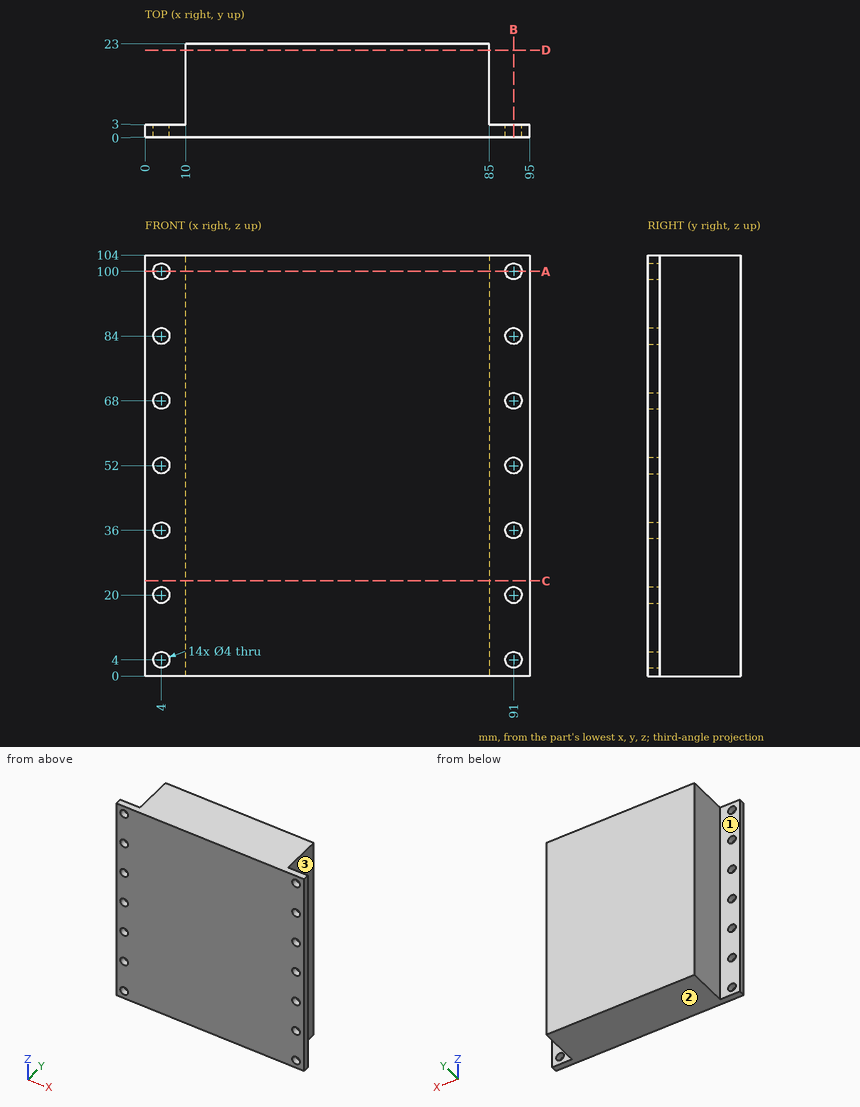
Job drawing, mm, ordinate dimensions from the low corner. One solid piece. A direction names the side the tool comes from. Coordinates: 2 decimals unless noted, no trailing zeros. Order: outer loops, then holes, each group sorted by start corner. A loop starts at its lowest first (then second) coordinate and runs counter-clockwise, first axis right, second up. Notation, with made-up numbers: (4, 21.5) - (16, 21.5) arc R26 cw to (16, 55.5) - close; hole circle Ø5 at (39, 67). An arc over 180 degrees is marked (long way). Return JSON: item names as keys, results as strings. Group by question number.
1) Tool access for the marked faces 1, 2 and 3: list every direction of +Z, -Z, +X, -X, +Y, -Y with a clear straight run to the whole face (end or side of a thin tool).
2) Saw through at C-C, the plane z = 23.5. Write the cut outline in (x, y), plus the area to 4 significant figures.
3) Flat gauge pins, fed straight in: P1, Ø5, axis at x = 88.5, z = 62.5, coming from the +Y side; P2, Ø12, axis at y = 11, z = 46, coming from the -X side; P3, Ø3.5, axis at x = 91, z = 52, coming from the +Y side; P4, Ø10, axis at y = 15.5, z = 34, coming from the +X side. Where does each tip first touch, or does it go through?
4) Saw through at B-B, the plane x = 91. Count the separate pieces of the cut face and the enclosed holes in it, plus the area to 3 significant figures.
5) Saw through at A-A, the plane z = 100. Write the cut outline in (x, y).
6) Saw through at D-D, the plane y = 21.5. Write the cut outline in (x, z).
7) Probe line 1 (X direction, y = 2.4, z = 4); line 2 (X direction, y = 9.25, z = 41.5); line 3 (Y direction, x = 6, z = 10). List the from-to ranges inside material, lowest first. Write a range as from..to.
Values found:
{
 "1": {"face 1": "+Z, -Z, -X, +Y", "face 2": "-Z, +X, -X, +Y, -Y", "face 3": "+Z, -Z, +X, +Y"},
 "2": {"outline": "(0, 0) - (95, 0) - (95, 3) - (85, 3) - (85, 23) - (10, 23) - (10, 3) - (0, 3) - close", "area": "1,785 mm²"},
 "3": {"P1": "stops at y = 3", "P2": "stops at x = 10", "P3": "passes through", "P4": "stops at x = 85"},
 "4": {"separate pieces": "8", "enclosed holes": "0", "area": "228 mm²"},
 "5": {"outline": "(0, 0) - (2, 0) - (2, 3) - (0, 3) - close; (6, 0) - (89, 0) - (89, 3) - (85, 3) - (85, 23) - (10, 23) - (10, 3) - (6, 3) - close; (93, 0) - (95, 0) - (95, 3) - (93, 3) - close"},
 "6": {"outline": "(10, 0) - (85, 0) - (85, 104) - (10, 104) - close"},
 "7": {"line 1": "x = 0..2, 6..89, 93..95", "line 2": "x = 10..85", "line 3": "y = 0..3"}
}
